from build123d import *

# Parameters (mm, degrees)
SURFACE_EXTRUDE1_1_DEPTH = 2500
THICKEN1_T1              = 3
BOSS_EXTRUDE1_REACH      = 2515.396
SKETCH2_W                = 29.660018132
SKETCH2_H                = 2


with BuildPart() as body_1:
    # Surface-Extrude1: a surface, the sketch's curves swept straight by 2500 mm
    with BuildLine(Plane.XY, mode=Mode.PRIVATE) as surface_extrude1_1_path:
        Line((-30, 257.405882212), (-30, 122.405882212))
        ThreePointArc((-30, 122.405882212), (-22.390634553, 59.391598117), (0, 0))
    surface_extrude1_1 = Shell.extrude(surface_extrude1_1_path.wire(), (0 * SURFACE_EXTRUDE1_1_DEPTH, 0 * SURFACE_EXTRUDE1_1_DEPTH, 1 * SURFACE_EXTRUDE1_1_DEPTH))
    add(Solid.thicken(surface_extrude1_1, THICKEN1_T1))

    # Sketch2 → Boss-Extrude1 (add, up to next)
    with BuildSketch(Plane(origin=(0, 257.405882212, 0), x_dir=(1, 0, 0), z_dir=(0, 1, 0)), mode=Mode.PRIVATE) as boss_extrude1_sk1:
        with Locations((-12.169990934, -2475)):
            Rectangle(SKETCH2_W, SKETCH2_H)
    boss_extrude1_tool1 = extrude(boss_extrude1_sk1.sketch, amount=-BOSS_EXTRUDE1_REACH, mode=Mode.PRIVATE) - body_1.part
    # Sketch2 → Boss-Extrude1 (add, up to next)
    with BuildSketch(Plane(origin=(0, 257.405882212, 0), x_dir=(1, 0, 0), z_dir=(0, 1, 0)), mode=Mode.PRIVATE) as boss_extrude1_sk2:
        with Locations((-12.169990934, -1985)):
            Rectangle(SKETCH2_W, SKETCH2_H)
    boss_extrude1_tool2 = extrude(boss_extrude1_sk2.sketch, amount=-BOSS_EXTRUDE1_REACH, mode=Mode.PRIVATE) - body_1.part
    # Sketch2 → Boss-Extrude1 (add, up to next)
    with BuildSketch(Plane(origin=(0, 257.405882212, 0), x_dir=(1, 0, 0), z_dir=(0, 1, 0)), mode=Mode.PRIVATE) as boss_extrude1_sk3:
        with Locations((-12.169990934, -1495)):
            Rectangle(SKETCH2_W, SKETCH2_H)
    boss_extrude1_tool3 = extrude(boss_extrude1_sk3.sketch, amount=-BOSS_EXTRUDE1_REACH, mode=Mode.PRIVATE) - body_1.part
    # Sketch2 → Boss-Extrude1 (add, up to next)
    with BuildSketch(Plane(origin=(0, 257.405882212, 0), x_dir=(1, 0, 0), z_dir=(0, 1, 0)), mode=Mode.PRIVATE) as boss_extrude1_sk4:
        with Locations((-12.169990934, -1005)):
            Rectangle(SKETCH2_W, SKETCH2_H)
    boss_extrude1_tool4 = extrude(boss_extrude1_sk4.sketch, amount=-BOSS_EXTRUDE1_REACH, mode=Mode.PRIVATE) - body_1.part
    # Sketch2 → Boss-Extrude1 (add, up to next)
    with BuildSketch(Plane(origin=(0, 257.405882212, 0), x_dir=(1, 0, 0), z_dir=(0, 1, 0)), mode=Mode.PRIVATE) as boss_extrude1_sk5:
        with Locations((-12.169990934, -515)):
            Rectangle(SKETCH2_W, SKETCH2_H)
    boss_extrude1_tool5 = extrude(boss_extrude1_sk5.sketch, amount=-BOSS_EXTRUDE1_REACH, mode=Mode.PRIVATE) - body_1.part
    # Sketch2 → Boss-Extrude1 (add, up to next)
    with BuildSketch(Plane(origin=(0, 257.405882212, 0), x_dir=(1, 0, 0), z_dir=(0, 1, 0)), mode=Mode.PRIVATE) as boss_extrude1_sk6:
        with Locations((-12.169990934, -25)):
            Rectangle(SKETCH2_W, SKETCH2_H)
    boss_extrude1_tool6 = extrude(boss_extrude1_sk6.sketch, amount=-BOSS_EXTRUDE1_REACH, mode=Mode.PRIVATE) - body_1.part
    add(boss_extrude1_tool1.solids().sort_by_distance((-12.169991, 257.405882, 2475))[0])
    add(boss_extrude1_tool2.solids().sort_by_distance((-12.169991, 257.405882, 1985))[0])
    add(boss_extrude1_tool3.solids().sort_by_distance((-12.169991, 257.405882, 1495))[0])
    add(boss_extrude1_tool4.solids().sort_by_distance((-12.169991, 257.405882, 1005))[0])
    add(boss_extrude1_tool5.solids().sort_by_distance((-12.169991, 257.405882, 515))[0])
    add(boss_extrude1_tool6.solids().sort_by_distance((-12.169991, 257.405882, 25))[0])


solid = body_1.part
Here's how the part is built. I have some questions about the finished solid (model axes, mm). A direction names the side the tool comes from. Round coordinates to 2 decimals unless told otherwise and drop trailing zeros. Order: outer loops, then holes, each group sorted by start corner. A loop starts at its lowest first (then second) coordinate and runs counter-clockwise, first axis right, second up. Notation, with made-up numbers: M -21.75,74 L 2.25,74 A24 cw 2.25,103 Z; hole C -13.5,-35 d2. An arc over 180 degrees is marked long. Return JSON: item names as keys, results as strings. Group by question number.
1. If we section it at A-A on z = 849: List the corners of the cut face in (x, y) for me, then the cut area to 3 significant figures.
2. If we section it at B-B on y = 171: List the corners of the cut face in (x, z) for me.
3. I'm going to push flat-ended pins straight in: pin 1 Ø10 at (x, y) = (-3.5, 27.5) entering from +Z; pin 2 Ø12 at (y, z) = (211, 1468.5) entering from +X. Where does each tip first touch, or does it pass through?
4. Please list where these lines run through material, in increasing order: probe 1 along Z at (x, y) = (-13, 139); probe 2 along X at (y, z) = (215, 636); probe 3 along X at (y, z) = (57.5, 246).
5. On a 3-axis mill with a long thin cutter (end or side, diameter ignored), from which of +Z, -Z, +X, -X, +Y, -Y can I reach the whole of each face in a straight line? I mean faces 4 (the face through (-27, 191, 1247)), 5 (the face through (-30, 191, 1232)). Say none if no direction works.
6. If we section it at C-C on x = -13.5: List the corners of the cut face in (y, z) for me.
7. If we mould it in two halves opening along Z, with no side actions, what happens to faces 1 (the face through (-19.685, 60.961, 1246.584)), 2 (the face through (-19.685, 60.961, 756.584)), 3 (the face through (-22.6, 60.26, 1232.5))? For each: pulls with the +Z half, pulls with the -Z half, needs draft (parallel to the pull), parting line crosses it, or undercut.
Reply:
{
 "1": {"outline": "M -30,122.41 A264.72 ccw 0,0 L 2.66,1.39 A261.72 cw -27,122.41 L -27,257.41 L -30,257.41 Z", "area": "785 mm^2"},
 "2": {"outline": "M -30,0 L -27,0 L -27,24 L 2.66,24 L 2.66,26 L -27,26 L -27,514 L 2.66,514 L 2.66,516 L -27,516 L -27,1004 L 2.66,1004 L 2.66,1006 L -27,1006 L -27,1494 L 2.66,1494 L 2.66,1496 L -27,1496 L -27,1984 L 2.66,1984 L 2.66,1986 L -27,1986 L -27,2474 L 2.66,2474 L 2.66,2476 L -27,2476 L -27,2500 L -30,2500 Z"},
 "3": {"pin 1": "z = 2476", "pin 2": "x = -27"},
 "4": {"probe 1": "24 to 26, 514 to 516, 1004 to 1006, 1494 to 1496, 1984 to 1986, 2474 to 2476", "probe 2": "-30 to -27", "probe 3": "-21.92 to -18.82"},
 "5": {"face 4": "+X, +Y", "face 5": "+Z, -Z, -X, +Y, -Y"},
 "6": {"outline": "M 30.41,0 L 39.43,0 L 39.43,24 L 257.41,24 L 257.41,26 L 39.43,26 L 39.43,514 L 257.41,514 L 257.41,516 L 39.43,516 L 39.43,1004 L 257.41,1004 L 257.41,1006 L 39.43,1006 L 39.43,1494 L 257.41,1494 L 257.41,1496 L 39.43,1496 L 39.43,1984 L 257.41,1984 L 257.41,1986 L 39.43,1986 L 39.43,2474 L 257.41,2474 L 257.41,2476 L 39.43,2476 L 39.43,2500 L 30.41,2500 Z"},
 "7": {"face 1": "undercut", "face 2": "undercut", "face 3": "needs draft"}
}
